The listing builds one solid part. Answer for the finished solid, in the listing's coordinates (mm). Give positions to 0.01 mm unless a question says otherwise; leave off trailing zeros. Write each loop counter-clockwise with the first axis right and the second up, starting at its lowest first coordinate (ties: lowest second). Pieces come first, ordered by that corner, then holes. Notation, with made-up numbers: M -30,48 L 29,48 A10 cw 29,57 Z; hole C 72.25,22 d7. An arc over 180 degrees is marked long. Return JSON: item names as keys, results as strings.
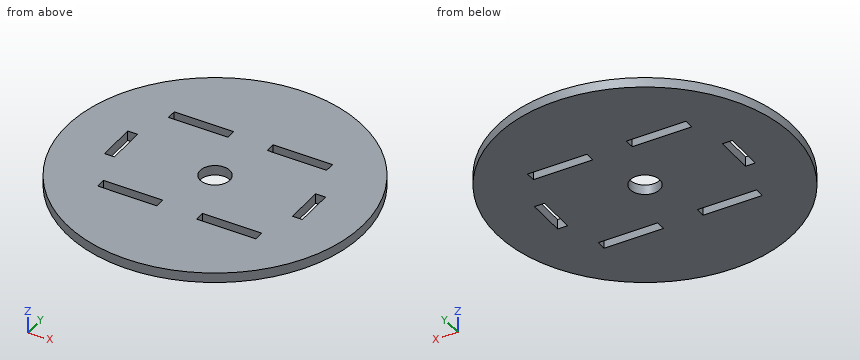
from build123d import *

# Parameters (mm, degrees)
SKETCH1_R           = 47.625
SKETCH1_R_2         = 4.7625
BOSS_EXTRUDE1_DEPTH = 3.175
SKETCH3_W           = 19.05
SKETCH3_H           = 3.175
CUT_EXTRUDE2_DEPTH  = 3.175


with BuildPart() as part:
    # Sketch1 → Boss-Extrude1 (new body)
    with BuildSketch(Plane.XY):
        Circle(SKETCH1_R)
        Circle(SKETCH1_R_2, mode=Mode.SUBTRACT)
    extrude(amount=BOSS_EXTRUDE1_DEPTH)

    # Sketch3 → Cut-Extrude2 (cut)
    with BuildSketch(Plane.XY):
        Polygon((-28.575, 0), (-28.575, -6.35), (-31.75, -6.35), (-31.75, 6.35), (-28.575, 6.35), align=None)
        Polygon((31.75, 0), (31.75, 6.35), (28.575, 6.35), (28.575, -6.35), (31.75, -6.35), align=None)
        with Locations((15.875, 19.3675)):
            Rectangle(SKETCH3_W, SKETCH3_H)
        with Locations((-15.875, 19.3675)):
            Rectangle(SKETCH3_W, SKETCH3_H)
        with Locations((-15.875, -19.3675)):
            Rectangle(SKETCH3_W, SKETCH3_H)
        with Locations((15.875, -19.3675)):
            Rectangle(SKETCH3_W, SKETCH3_H)
    extrude(amount=CUT_EXTRUDE2_DEPTH, mode=Mode.SUBTRACT)


solid = part.part
Item 1: A cutting plane is placed at D-D, the plane x = -21. Write down the section's boundary in (y, z) (3 decimals), plus the area to 3 significant figures.
Geometry results:
{"outline": "M -42.745,0 L -20.955,0 L -20.955,3.175 L -42.745,3.175 Z; M -17.78,0 L 17.78,0 L 17.78,3.175 L -17.78,3.175 Z; M 20.955,0 L 42.745,0 L 42.745,3.175 L 20.955,3.175 Z", "area": "251 mm2"}
Item 2: A cutting plane is placed at B-B, the plane y = 0. Count the separate pieces of the cut face and the enclosed holes in it, plus the area to 3 significant figures.
Geometry results:
{"separate pieces": "4", "enclosed holes": "0", "area": "252 mm2"}
Item 3: A cutting plane is placed at A-A, the plane x = 0. Write down the section's boundary in (y, z) (1 decimal), plus the area to 3 significant figures.
Geometry results:
{"outline": "M -47.6,0 L -4.8,0 L -4.8,3.2 L -47.6,3.2 Z; M 4.8,0 L 47.6,0 L 47.6,3.2 L 4.8,3.2 Z", "area": "272 mm2"}
Item 4: Given pin 1 Ø1 at (x, z) = (-30.5, 1.5) entering from +Y; pin 2 Ø1 at (x, z) = (-18, 2) entering from -Y; pin 3 Ø1 at (y, z) = (-20, 2) entering from +X; pin 4 Ø1.5 at (x, y) = (-25.5, 10) entering from -Z, each flat-ended and moving along its own axis, determine where each tip first touches the part or whether it passes through.
Geometry results:
{"pin 1": "stops at y = 36.99", "pin 2": "stops at y = -44.29", "pin 3": "stops at x = 43.45", "pin 4": "stops at z = 0"}
Item 5: Find the intervals of material crossed by line 1 (Y direction, x = 0, z = 1.15) (1 decimal); line 2 (Y direction, x = -23.5, z = 2.15) (3 decimals); line 3 (Y direction, x = -10, z = 0.2) (3 decimals), in increasing order.
Geometry results:
{"line 1": "y = -47.6 to -4.8, 4.8 to 47.6", "line 2": "y = -41.423 to -20.955, -17.78 to 17.78, 20.955 to 41.423", "line 3": "y = -46.563 to -20.955, -17.78 to 17.78, 20.955 to 46.563"}
